Autodesk Inventor part; units mm, degrees
ref_plane "YZ Plane" through (0, 0, 0) normal (1, 0, 0) x (0, 1, 0)
ref_plane "XZ Plane" through (0, 0, 0) normal (0, 1, 0) x (-1, 0, 0)
ref_plane "XY Plane" through (0, 0, 0) normal (0, 0, 1) x (1, 0, 0)
sketch "Эскиз1" plane through (0, 0, 0) normal (0, 0, 1) x (1, 0, 0)
  arc A0 (19.3, -19.3) -> (22.3, -16.3) centre (19.3, -16.3) ccw
  line L0 (19.3, -19.3) -> (-19.3, -19.3)
  arc A1 (-22.3, -16.3) -> (-19.3, -19.3) centre (-19.3, -16.3) ccw
  line L1 (-22.3, -16.3) -> (-22.3, 16.3)
  arc A2 (-19.3, 19.3) -> (-22.3, 16.3) centre (-19.3, 16.3) ccw
  line L2 (-19.3, 19.3) -> (19.3, 19.3)
  arc A3 (22.3, 16.3) -> (19.3, 19.3) centre (19.3, 16.3) ccw
  line L3 (22.3, 16.3) -> (22.3, -16.3)
  circle A4 centre (-19.3, 16.3) radius 2 construction
  circle A5 centre (19.3, 16.3) radius 2 construction
  circle A6 centre (19.3, -16.3) radius 2 construction
  circle A7 centre (-19.3, -16.3) radius 2 construction
  arc A8 (14.15, 1.4869) -> (1.4869, 14.15) centre (9.15, 9.15) ccw
  line L4 (1.4869, 14.15) -> (-1.4869, 14.15)
  arc A9 (-1.4869, 14.15) -> (-14.15, 1.4869) centre (-9.15, 9.15) ccw
  line L5 (-14.15, 1.4869) -> (-14.15, -1.4869)
  arc A10 (-14.15, -1.4869) -> (-1.4869, -14.15) centre (-9.15, -9.15) ccw
  line L6 (-1.4869, -14.15) -> (1.4869, -14.15)
  arc A11 (1.4869, -14.15) -> (14.15, -1.4869) centre (9.15, -9.15) ccw
  line L7 (14.15, -1.4869) -> (14.15, 1.4869)
  line L8 (-9.15, 9.15) -> (-18.3, 9.15) construction
  line L9 (-22.3, 0) -> (22.3, 0) construction
  line L10 (0, 19.3) -> (0, -19.3) construction
  line L11 (-9.15, -9.15) -> (-18.3, -9.15) construction
  line L12 (-9.15, 9.15) -> (-9.15, 18.3) construction
  line L13 (9.15, 9.15) -> (9.15, 18.3) construction
  line L14 (-18.3, 9.15) -> (-18.3, -9.15)
  line L15 (-9.15, 18.3) -> (9.15, 18.3)
  line L16 (-9.15, -18.3) -> (9.15, -18.3)
  line L17 (18.3, 9.15) -> (18.3, -9.15)
  line L18 (-18.3, 9.15) -> (-18.3, 4.15) construction
  line L19 (-18.3, -9.15) -> (-18.3, -4.15) construction
  line L20 (-18.3, 4.15) -> (-21.3, 4.15)
  line L21 (-21.3, 4.15) -> (-21.3, -4.15)
  line L22 (-21.3, -4.15) -> (-18.3, -4.15)
  line L23 (-18.3, -4.15) -> (-18.3, 4.15)
  line L24 (18.3, 4.15) -> (21.3, 4.15)
  line L25 (21.3, 4.15) -> (21.3, -4.15)
  line L26 (21.3, -4.15) -> (18.3, -4.15)
  line L27 (18.3, -4.15) -> (18.3, 4.15)
  circle A12 centre (-19.3, 16.3) radius 1.5
  circle A13 centre (19.3, 16.3) radius 1.5
  circle A14 centre (19.3, -16.3) radius 1.5
  circle A15 centre (-19.3, -16.3) radius 1.5
  dimension "d0" = 5
  dimension "d1" = 5
  dimension "d2" = 3
  dimension "d3" = 8.3
  dimension "d4" = 3
  dimension "d5" = 3
  dimension "d6" = 3
  dimension "d7" = 3
extrude "Выдавливание1" add sketch "Эскиз1" along normal blind 6.4 contours L0 A1 L1 A2 L2 A3 L3 A0 | L7 A11 L6 A10 L5 A9 L4 A8 | A8 L17 A11 L7 | A8 L4 A9 L15 | L24 L25 L26 L17 | L16 A10 L6 A11 | A9 L5 A10 L14 | L14 L22 L21 L20
extrude "Выдавливание2" cut sketch "Эскиз1" along normal blind 4.4 contours L7 A11 L6 A10 L5 A9 L4 A8 | A8 L17 A11 L7 | A8 L4 A9 L15 | L24 L25 L26 L17 | L16 A10 L6 A11 | A9 L5 A10 L14 | L14 L22 L21 L20
chamfer "Фаска1" distance 2 angle 45 4 edges at (17.8, 16.3, 6.4) (17.8, -16.3, 6.4) (-20.8, -16.3, 6.4) (-20.8, 16.3, 6.4)
fillet "Сопряжение1" radius 2 2 edges at (-21.3, 0, 4.4) (21.3, 0, 4.4)
properties part number "akkum_cap_bms"
Could you check a few things on this model? Use its own coordinates, in mm. A direction names the side the tool comes from. Give positions to 0.01 mm unless a question says otherwise; leave off trailing zeros. Loops run counter-clockwise (first coordinate to the right, second up) from the corner with the lowest first, then second, coordinate; pieces in that order, holes last. Notation, with made-up numbers: (30, 61.5) - (44, 61.5) arc R24 ccw to (44, 72.5) - close; hole circle Ø8 at (-29.5, 68). An arc over 180 degrees is marked (long way). Use one line per item in the form item = value.
1. On a 3-axis mill with a long thin cutter (end or side, diameter ignored), from which of +Z, -Z, +X, -X, +Y, -Y can I reach the whole of each face in a straight line? I mean faces 1 (the face through (20, -4.15, 2)), 2 (the face through (-19.625, -14.836, 2.169)). Say none if no direction works.
Response values:
face_1 = -Z
face_2 = +Z, -Z
2. I'm going to push flat-ended pins straight in: pin 1 Ø3.5 at (x, y) = (-19.3, -16.3) entering from +Z; pin 2 Ø1.5 at (x, z) = (-19.5, 2) entering from +Y; pin 3 Ø4 at (x, y) = (19.3, 16.3) entering from +Z. Where does each tip first touch, or does it pass through?
Response values:
pin_1 = 4.65
pin_2 = 19.3
pin_3 = 4.9
3. I want a section at B-B (x = 6). Please give me the cut outline in (y, z).
Response values:
outline = (-19.3, 0) - (-18.3, 0) - (-18.3, 4.4) - (18.3, 4.4) - (18.3, 0) - (19.3, 0) - (19.3, 6.4) - (-19.3, 6.4) - close
4. I need wall thicknesses on probe 1 along Y at (x, z) = (-19.3, 2.4); probe 2 along Y at (x, z) = (5, 4.25); probe 3 along X at (y, z) = (16, 5.5). Which ranges of each line are inside material? Lowest first, please.
Response values:
probe_1 = -19.3 to -17.8, -14.8 to -4.15, 4.15 to 14.8, 17.8 to 19.3
probe_2 = -19.3 to -18.3, 18.3 to 19.3
probe_3 = -22.3 to -21.88, -16.72 to 16.72, 21.88 to 22.3
5. I want a section at D-D (y = 7). Please give me the cut outline in (x, z), and give its area (3 significant figures).
Response values:
outline = (-22.3, 0) - (-18.3, 0) - (-18.3, 4.4) - (18.3, 4.4) - (18.3, 0) - (22.3, 0) - (22.3, 6.4) - (-22.3, 6.4) - close
area = 124 mm²
6. I want a section at C-C (z = 1). Please give me the cut outline in (x, y).
Response values:
outline = (-22.3, -16.3) arc R3 ccw to (-19.3, -19.3) - (19.3, -19.3) arc R3 ccw to (22.3, -16.3) - (22.3, 16.3) arc R3 ccw to (19.3, 19.3) - (-19.3, 19.3) arc R3 ccw to (-22.3, 16.3) - close; hole (-21.3, -4.15) - (-18.3, -4.15) - (-18.3, -9.15) arc R9.15 ccw to (-9.15, -18.3) - (9.15, -18.3) arc R9.15 ccw to (18.3, -9.15) - (18.3, -4.15) - (21.3, -4.15) - (21.3, 4.15) - (18.3, 4.15) - (18.3, 9.15) arc R9.15 ccw to (9.15, 18.3) - (-9.15, 18.3) arc R9.15 ccw to (-18.3, 9.15) - (-18.3, 4.15) - (-21.3, 4.15) - close; hole circle Ø3 at (-19.3, -16.3); hole circle Ø3 at (-19.3, 16.3); hole circle Ø3 at (19.3, -16.3); hole circle Ø3 at (19.3, 16.3)
7. Thinking about a two-plate mould opening in Y: for faces 3 (the face through (-18.426, -14.93, 4.525)), 4 (the face through (0, 19.3, 3)), 5 (the face through (-21.4, -18.44, 2.91)), 6 (the face through (0, 0, 6.4)), which applies, released by +Y, released by -Y, zero draft, split by the parting line, or undercut?
Response values:
face_3 = undercut
face_4 = released by +Y
face_5 = released by -Y
face_6 = zero draft
8. I want a section at A-A (z = 5). Please give me the cut outline in (x, y), and give its area (3 significant figures).
Response values:
outline = (-22.3, -16.3) arc R3 ccw to (-19.3, -19.3) - (19.3, -19.3) arc R3 ccw to (22.3, -16.3) - (22.3, 16.3) arc R3 ccw to (19.3, 19.3) - (-19.3, 19.3) arc R3 ccw to (-22.3, 16.3) - close; hole circle Ø4.2 at (-19.3, -16.3); hole circle Ø4.2 at (-19.3, 16.3); hole circle Ø4.2 at (19.3, -16.3); hole circle Ø4.2 at (19.3, 16.3)
area = 1,660 mm²
